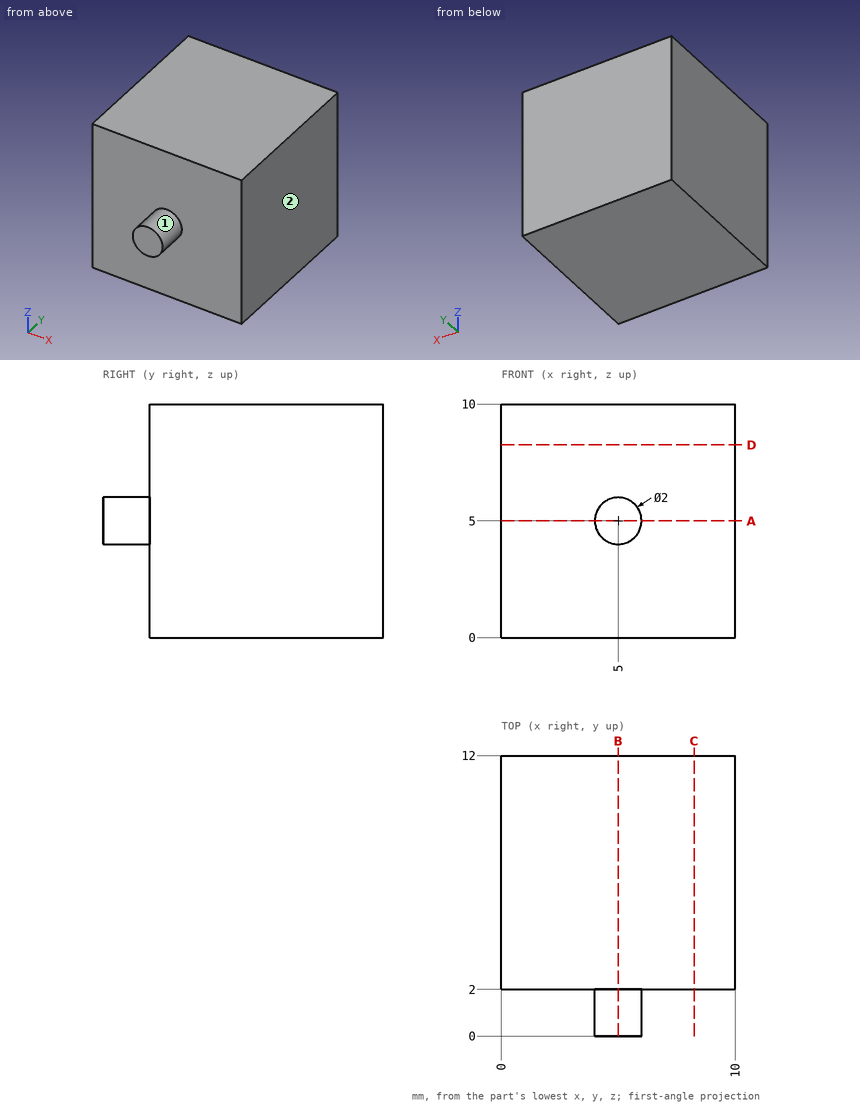
Job drawing, mm, ordinate dimensions from the low corner. One solid piece. A direction names the side the tool comes from. Round coordinates to 2 decimals unless told otherwise and drop trailing zeros. Loops run counter-clockwise (first coordinate to the right, second up) from the corner with the lowest first, then second, coordinate; pieces in that order, holes last.
Item 1: Cut at D-D, the plane z = 8.25. Give the cut face in (x, y), then the cut area to 3 significant figures.
Item 2: Cut at C-C, the plane x = 8.25. Give the cut face in (y, z).
Item 3: Cut at B-B, the plane x = 5. Give the cut face in (y, z).
Item 4: 3-axis set-ups, long thin cutter, end or side, ignore diameter. For the marked faces 1 and 2: which of +Z, -Z, +X, -X, +Y, -Y reach the whole face in a straight line?
Item 5: Drill centre lines: line 1 (Y direction, x = 2.5, z = 9); line 2 (Z direction, x = 4.5, y = 1.5). Where is each one in solid material? Low to high.
Item 6: Cut at A-A, the plane z = 5. Give the cut face in (x, y).
A:
1. outline: (0, 2) - (10, 2) - (10, 12) - (0, 12) - close
1. area: 100 mm2
2. outline: (2, 0) - (12, 0) - (12, 10) - (2, 10) - close
3. outline: (0, 4) - (2, 4) - (2, 0) - (12, 0) - (12, 10) - (2, 10) - (2, 6) - (0, 6) - close
4. face 1: -Y
4. face 2: +Z, -Z, +X, +Y, -Y
5. line 1: y = 2 to 12
5. line 2: z = 4.13 to 5.87
6. outline: (0, 2) - (4, 2) - (4, 0) - (6, 0) - (6, 2) - (10, 2) - (10, 12) - (0, 12) - close
